from build123d import *

# Parameters (mm, degrees)
IZIM1_W                     = 48
IZIM1_H                     = 36
IZIM1_W_2                   = 2.8
IZIM1_H_2                   = 2.8
Y_KSEKLIK_EKSTR_ZYON1_DEPTH = 10
IZIM2_R                     = 1.979898987
KES_EKSTR_ZYON2_DEPTH       = 10


with BuildPart() as part:
    # Çizim1 → Yükseklik-Ekstrüzyon1 (new body)
    with BuildSketch(Plane.XY):
        Rectangle(IZIM1_W, IZIM1_H)
        with Locations((-4, -8)):
            Rectangle(IZIM1_W_2, IZIM1_H_2, mode=Mode.SUBTRACT)
    extrude(amount=Y_KSEKLIK_EKSTR_ZYON1_DEPTH)

    # Çizim2 → Kes-Ekstrüzyon2 (cut)
    with BuildSketch(Plane.XY.offset(10)):
        with Locations((-4, -8)):
            Circle(IZIM2_R)
    extrude(amount=-KES_EKSTR_ZYON2_DEPTH, mode=Mode.SUBTRACT)


solid = part.part
Here's how the part is built. I have some questions about the finished solid (model axes, mm). Coordinates: 2 decimals unless noted, no trailing zeros. Write each loop counter-clockwise with the first axis right and the second up, starting at its lowest first coordinate (ties: lowest second). Pieces come first, ordered by that corner, then holes.
Item 1: I want a section at A-A on x = -4. Write out the boundary of the cut face in (y, z), and give its area (3 significant figures).
Item 2: If we mould it in two halves opening along Y, with no side actions, what happens to faces 1 (the cylindrical face through (-5.571, -9.205, 5.07)), 2 (the flat face through (0, -18, 5)), 3 (the flat face through (24, 0, 5))? For each: +Y half, -Y half, draft (parallel to the pull), parting line (faces both ways), or undercut.
Item 3: I want a section at B-B on y = -8. Write out the boundary of the cut face in (x, z).
Item 4: If I drill on line 1 (X direction, y = -8, z = 7.75); line 2 (Y direction, x = -4, z = 2.75); line 3 (X direction, y = -8.5, z = 3), over which ranges is the centre line in solid material (lowest first)?
Findings below:
1. outline: (-18, 0) - (-9.98, 0) - (-9.98, 10) - (-18, 10) - close; (-6.02, 0) - (18, 0) - (18, 10) - (-6.02, 10) - close
1. area: 320 mm2
2. face 1: undercut
2. face 2: -Y half
2. face 3: draft
3. outline: (-24, 0) - (-5.98, 0) - (-5.98, 10) - (-24, 10) - close; (-2.02, 0) - (24, 0) - (24, 10) - (-2.02, 10) - close
4. line 1: x = -24 to -5.98, -2.02 to 24
4. line 2: y = -18 to -9.98, -6.02 to 18
4. line 3: x = -24 to -5.92, -2.08 to 24
